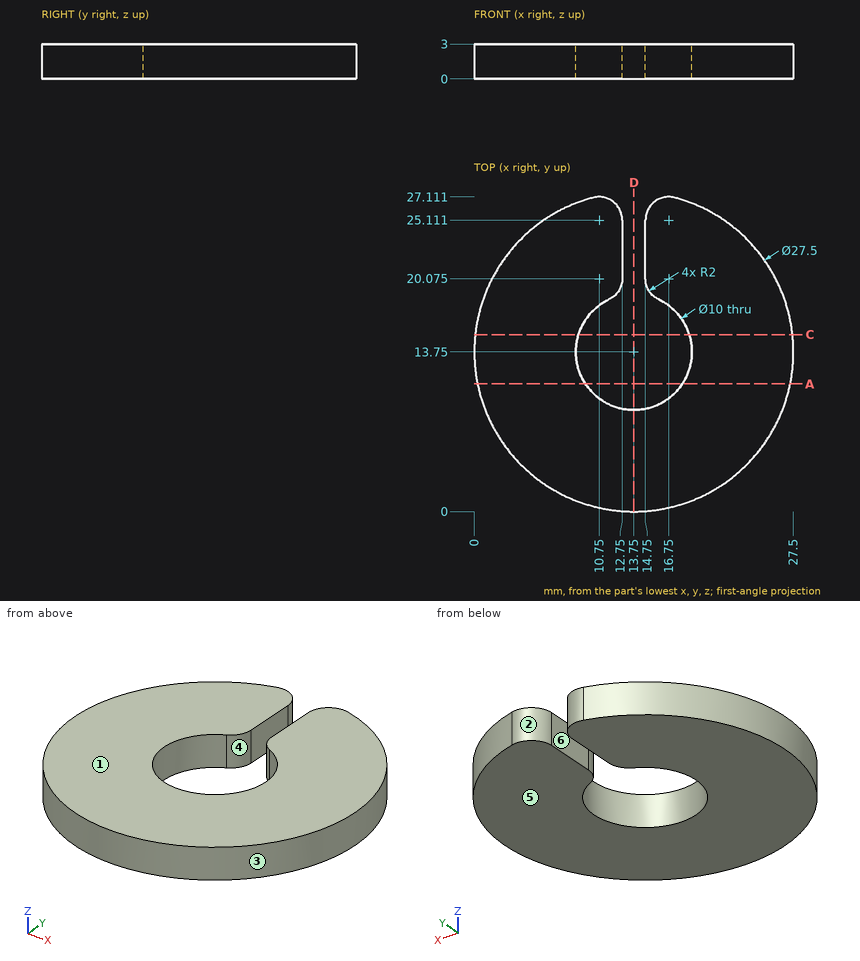
Here's the drawing with two shaded views (mm, measured from the low corner). I have some questions. A direction names the side the tool comes from. Coordinates: 2 decimals unless noted, no trailing zeros. Order: outer loops, then holes, each group sorted by start corner. A loop starts at its lowest first (then second) coordinate and runs counter-clockwise, first axis right, second up. Notation, with made-up numbers: (24.5, -18) -> (30.5, -18) arc R8 ccw to (30.5, -12) -> close; hole circle Ø10 at (20, 18.25). An arc over 180 degrees is marked (long way). One line per question, with ' | ' between items.
Q1. On a 3-axis mill with a long thin cutter (end or side, diameter ignored), from which of +Z, -Z, +X, -X, +Y, -Y can I reach the whole of each face in a straight line? I mean the marked faces 4, 5 and 6. Say none if no direction works.
Return value:
face 4: +Z, -Z | face 5: -Z, +X, -X, +Y, -Y | face 6: +Z, -Z, +Y
Q2. Imagine slicing it at C-C on y = 15.25. Please give me the cut outline in (x, z).
Return value:
outline: (0.08, 0) -> (8.98, 0) -> (8.98, 3) -> (0.08, 3) -> close; (18.52, 0) -> (27.42, 0) -> (27.42, 3) -> (18.52, 3) -> close
Q3. Imagine slicing it at D-D on x = 13.75. Please give me the cut outline in (y, z).
Return value:
outline: (0, 0) -> (8.75, 0) -> (8.75, 3) -> (0, 3) -> close
Q4. I'm going to push flat-ended pins straight in: P1, Ø1, axis at x = 19, y = 15, coming from the -Z side; P2, Ø1, axis at y = 18.5, z = 1, coming from the -X side; P3, Ø0.9, axis at y = 23.5, z = 1.5, coming from the +X side; P4, Ø1.5, axis at x = 10.5, z = 1, coming from the -Y side. Where does each tip first touch, or does it pass through?
Return value:
P1: z = 0 | P2: x = 0.67 | P3: x = 23.88 | P4: y = 0.23
Q5. Thinking about a two-plate mould opening in X: for the marked faces 1, 2 and 3, which applies, pulls with the +X half, pulls with the -X half, needs draft (parallel to the pull), parting line crosses it, or undercut?
Return value:
face 1: needs draft | face 2: undercut | face 3: parting line crosses it
Q6. Imagine slicing it at A-A on y = 11. Please give me the cut outline in (x, z) (1 decimal).
Return value:
outline: (0.3, 0) -> (9.6, 0) -> (9.6, 3) -> (0.3, 3) -> close; (17.9, 0) -> (27.2, 0) -> (27.2, 3) -> (17.9, 3) -> close
Q7. If I drill on L1, parallel to X at y = 16.5, z = 0.25 (1 decimal); L2, parallel to X at y = 10.5, z = 2.2; L3, parallel to Y at x = 16.5, z = 0.3 (1 decimal), over which ranges is the centre line in solid material (lowest first)?
Return value:
L1: 0.3 to 9.6, 17.9 to 27.2 | L2: 0.39 to 9.95, 17.55 to 27.11 | L3: 0.3 to 9.6, 17.9 to 27.1
